```python
from build123d import *

# Parameters (mm, degrees)
CYLINDER009_R     = 1.6
CYLINDER009_DEPTH = 20
CYLINDER008_R     = 1.6
CYLINDER008_DEPTH = 20
CYLINDER007_R     = 1.6
CYLINDER007_DEPTH = 20
CYLINDER006_R     = 1.6
CYLINDER006_DEPTH = 10
CYLINDER005_R     = 1.6
CYLINDER005_DEPTH = 10
CYLINDER004_R     = 1.6
CYLINDER004_DEPTH = 10
BOX002_W          = 11.5
BOX002_H          = 40
BOX002_DEPTH      = 4
BOX003_W          = 10
BOX003_H          = 40
BOX003_DEPTH      = 14
BOX001_W          = 17.5
BOX001_H          = 40
BOX001_DEPTH      = 2.75


with BuildPart() as cylinder009:
    # Cylinder009 → Cylinder009 (new body)
    with BuildSketch(Plane(origin=(50, 70, -5), x_dir=(1, 0, 0), z_dir=(0, 0, 1))):
        Circle(CYLINDER009_R)
    extrude(amount=CYLINDER009_DEPTH)


with BuildPart() as cylinder008:
    # Cylinder008 → Cylinder008 (new body)
    with BuildSketch(Plane(origin=(39, 70, -5), x_dir=(1, 0, 0), z_dir=(0, 0, 1))):
        Circle(CYLINDER008_R)
    extrude(amount=CYLINDER008_DEPTH)


with BuildPart() as cylinder007:
    # Cylinder007 → Cylinder007 (new body)
    with BuildSketch(Plane(origin=(39, 65, -5), x_dir=(1, 0, 0), z_dir=(0, 0, 1))):
        Circle(CYLINDER007_R)
    extrude(amount=CYLINDER007_DEPTH)


with BuildPart() as cylinder006:
    # Cylinder006 → Cylinder006 (new body)
    with BuildSketch(Plane(origin=(27, 65, -5), x_dir=(1, 0, 0), z_dir=(0, 0, 1))):
        Circle(CYLINDER006_R)
    extrude(amount=CYLINDER006_DEPTH)


with BuildPart() as cylinder005:
    # Cylinder005 → Cylinder005 (new body)
    with BuildSketch(Plane(origin=(27, 70, -5), x_dir=(1, 0, 0), z_dir=(0, 0, 1))):
        Circle(CYLINDER005_R)
    extrude(amount=CYLINDER005_DEPTH)


with BuildPart() as cylinder004:
    # Cylinder004 → Cylinder004 (new body)
    with BuildSketch(Plane(origin=(9, 70, -5), x_dir=(1, 0, 0), z_dir=(0, 0, 1))):
        Circle(CYLINDER004_R)
    extrude(amount=CYLINDER004_DEPTH)


with BuildPart() as cube002:
    # Box002 → Box002 (new body)
    with BuildSketch(Plane(origin=(27.5, 50, 0), x_dir=(1, 0, 0), z_dir=(0, 0, 1))):
        with Locations((5.75, 20)):
            Rectangle(BOX002_W, BOX002_H)
    extrude(amount=BOX002_DEPTH)


with BuildPart() as cube003:
    # Box003 → Box003 (new body)
    with BuildSketch(Plane(origin=(39, 50, 0), x_dir=(1, 0, 0), z_dir=(0, 0, 1))):
        with Locations((5, 20)):
            Rectangle(BOX003_W, BOX003_H)
    extrude(amount=BOX003_DEPTH)


with BuildPart() as cut005:
    # Box001 → Box001 (new body)
    with BuildSketch(Plane(origin=(10, 50, 0), x_dir=(1, 0, 0), z_dir=(0, 0, 1))):
        with Locations((8.75, 20)):
            Rectangle(BOX001_W, BOX001_H)
    extrude(amount=BOX001_DEPTH)

    # Fusion: union Cube002, Cube003
    add(cube002.part)
    add(cube003.part)

    # Cut: cut Cylinder004
    add(cylinder004.part, mode=Mode.SUBTRACT)

    # Cut001: cut Cylinder005
    add(cylinder005.part, mode=Mode.SUBTRACT)

    # Cut002: cut Cylinder006
    add(cylinder006.part, mode=Mode.SUBTRACT)

    # Cut003: cut Cylinder007
    add(cylinder007.part, mode=Mode.SUBTRACT)

    # Cut004: cut Cylinder008
    add(cylinder008.part, mode=Mode.SUBTRACT)

    # Cut005: cut Cylinder009
    add(cylinder009.part, mode=Mode.SUBTRACT)


solid = cut005.part
```
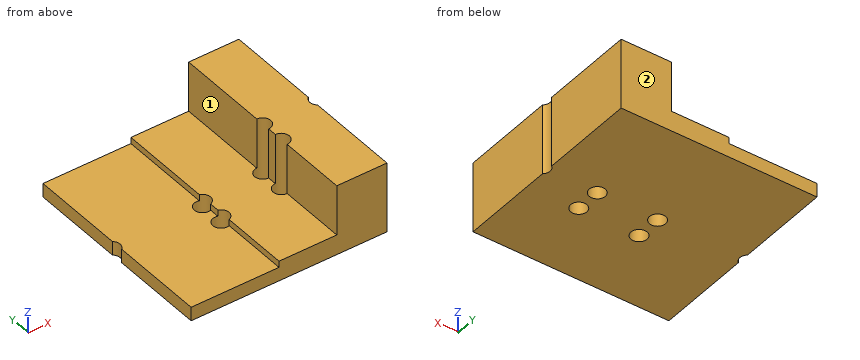
CAD build for the part. Positions are in the model's coordinates, mm. Face numbers are marked on the shaded views. A direction names the side the tool comes from. Round coordinates to 2 decimals unless told otherwise and drop trailing zeros. Write each loop counter-clockwise with the first axis right and the second up, starting at its lowest first coordinate (ties: lowest second). Pieces come first, ordered by that corner, then holes.
Item 1: Band-saw the part on A-A on x = 27. Write the cut outline in (y, z), then the cut area to 3 significant figures.
Filled in:
outline: (50, 0) - (63.4, 0) - (63.4, 2.75) - (50, 2.75) - close; (66.6, 0) - (68.4, 0) - (68.4, 2.75) - (66.6, 2.75) - close; (71.6, 0) - (90, 0) - (90, 2.75) - (71.6, 2.75) - close
area: 92.4 mm2
Item 2: Drill centre lines: L1, parallel to Y at x = 27, z = 2; L2, parallel to X at y = 65, z = 2.6; L3, parallel to X at y = 65, z = 3. Where is each one in solid material? Low to high.
Filled in:
L1: y = 50 to 63.4, 66.6 to 68.4, 71.6 to 90
L2: x = 10 to 25.4, 28.6 to 37.4, 40.6 to 49
L3: x = 28.6 to 37.4, 40.6 to 49
Item 3: Tool access for the marked faces 1 and 2: list every direction of +Z, -Z, +X, -X, +Y, -Y with a clear straight run to the whole face (end or side of a thin tool).
Filled in:
face 1: +Z, -X, +Y, -Y
face 2: +Z, -Z, +X, -X, +Y
Item 4: Band-saw the part on D-D on y = 87.5. Write the cut outline in (x, z).
Filled in:
outline: (10, 0) - (49, 0) - (49, 14) - (39, 14) - (39, 4) - (27.5, 4) - (27.5, 2.75) - (10, 2.75) - close
Item 5: Drop flat-ended pins along their axis: pin 1 Ø1.4 at (y, z) = (67.5, 3.5) entering from -X; pin 2 Ø4 at (x, y) = (27, 70) entering from +Z; pin 3 Ø5.5 at (x, y) = (21, 66.5) entering from +Z. Give the stop position or say it passes through.
Filled in:
pin 1: stops at x = 27.5
pin 2: stops at z = 4
pin 3: stops at z = 2.75
Item 6: Band-saw the part on B-B on y = 65. Write the cut outline in (x, z), then the cut area to 3 significant figures.
Filled in:
outline: (10, 0) - (25.4, 0) - (25.4, 2.75) - (10, 2.75) - close; (28.6, 0) - (37.4, 0) - (37.4, 4) - (28.6, 4) - close; (40.6, 0) - (49, 0) - (49, 14) - (40.6, 14) - close
area: 195 mm2
Item 7: Band-saw the part on C-C on z = 12. Write the cut outline in (x, y), then the cut area to 3 significant figures.
Filled in:
outline: (39, 50) - (49, 50) - (49, 68.75) arc R1.6 cw to (49, 71.25) - (49, 90) - (39, 90) - (39, 71.6) arc R1.6 cw to (39, 68.4) - (39, 66.6) arc R1.6 cw to (39, 63.4) - close
area: 391 mm2
